Build history of the part. All positions in model axes, mm. Face numbers are marked on the shaded views. A direction names the side the tool comes from. Round coordinates to 2 decimals unless told otherwise and drop trailing zeros. Order: outer loops, then holes, each group sorted by start corner. A loop starts at its lowest first (then second) coordinate and runs counter-clockwise, first axis right, second up. Notation, with made-up numbers: M 88,54 L 94,54 A14 cw 94,71 Z; hole C 35.25,4.25 d2. An arc over 180 degrees is marked long. One line per item, written item: value. Start each with the question number.
Item 1: Pin check, flat tips, straight feed: pin 1 (1.5 mm diameter, centred on x = 0, y = -19, fed in from +Z) (3 decimals); pin 2 (1.3 mm diameter, centred on y = -19, z = 10.5, fed in from -X); pin 3 (3 mm diameter, centred on x = 4.5, y = 1.25, fed in from -Z); pin 4 (3.5 mm diameter, centred on y = -18.5, z = 7.5, fed in from +X). Stop position of each tip, or through.
Item 2: Band-saw the part on B-B, the plane x = 0. Write the cut outline in (y, z).
Item 3: Probe L1, parallel to Y at x = 0, z = 20; L2, parallel to X at y = 1.25, z = 12.25; L3, parallel to Y at x = -1, z = 7.25. List the from-to ranges inside material, lowest first.
Item 4: Band-saw the part on D-D, the plane z = 19. Write the cut outline in (x, y), then the cut area to 3 significant figures.
Item 5: Two-plate mould, pull along X, no slides. Class the marked faces 5, 6, 7 and 8: +X half, -X half, draft (parallel to the pull), parting line (faces both ways), or undercut.
Item 6: Band-saw the part on C-C, the plane y = 1.25. Write the cut outline in (x, z), then the cut area to 3 significant figures.
Item 7: Tool access for the marked faces 1, 2, 3 and 4: list every direction of +Z, -Z, +X, -X, +Y, -Y with a clear straight run to the whole face (end or side of a thin tool).
Item 8: Band-saw the part on A-A, the plane z = 16. Write the cut outline in (x, y), then the cut area to 3 significant figures.
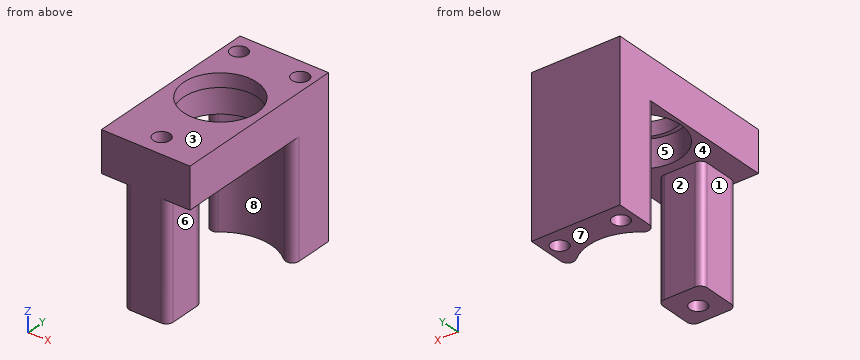
Autodesk Inventor part; units mm, degrees
ref_plane "YZ Plane" through (0, 0, 0) normal (1, 0, 0) x (0, 1, 0)
ref_plane "XZ Plane" through (0, 0, 0) normal (0, 1, 0) x (-1, 0, 0)
ref_plane "XY Plane" through (0, 0, 0) normal (0, 0, 1) x (1, 0, 0)
sketch "Sketch1" plane through (0, 0, 0) normal (0, 0, 1) x (1, 0, 0)
  line L0 (-6.5, 4) -> (6.5, 4)
  line L1 (6.5, 4) -> (6.5, -4)
  line L2 (6.5, -4) -> (-6.5, -4)
  line L3 (-6.5, -4) -> (-6.5, 4)
  line L4 (-6.5, 4) -> (6.5, -4) construction
  line L5 (6.5, 4) -> (-6.5, -4) construction
  point P0 (0, 0)
  point P1 (4.5, 1.25)
  point P2 (-4.5, 1.25)
  dimension "d0" = 13
  dimension "d1" = 8
  dimension "d64" = 2.75
  dimension "d65" = 2
  dimension "d66" = 2.75
  dimension "d67" = 2
extrude "Extrusion1" add sketch "Sketch1" along normal blind 48
hole "Hole1" at (-4.5, 1.25, 0) at (4.5, 1.25, 0) direction (0, 0, 1) diameter 2.459 end through all
sketch "Sketch6" plane through (-6.5, -4, 0) normal (0, -1, 0) x (1, 0, 0)
  line L0 (0.2, 0) -> (0, 0)
  line L1 (12.8, 0) -> (12.8, 36.9748)
  line L2 (0, 0) -> (12.8, 0)
  line L3 (12.8, 0) -> (12.8, 17)
  line L4 (12.8, 17) -> (0, 17)
  line L5 (0, 17) -> (0, 0)
  line L6 (13, 0) -> (13, 48)
  line L7 (0, 17) -> (13, 17)
  line L8 (13, 17) -> (13, 23)
  line L9 (13, 23) -> (0, 23)
  line L10 (0, 23) -> (0, 17)
  point P0 (6.5, 0)
  point P1 (12.8, 36.8338)
  point P2 (13, 36.8338)
  point P3 (13, 37.0101)
  dimension "d60" = 17
  dimension "d61" = 6
extrude "Extrusion3" add sketch "Sketch6" along normal blind 18 contours L10 L9 L1 L4 | L1 L9 L6 L7
sketch "Sketch7" plane through (6.5, -4, 17) normal (0, 0, -1) x (-1, 0, 0)
  line L0 (13, 8) -> (0, 8)
  circle A0 centre (6.5, -4) radius 6
  point P0 (6.5, 4)
  dimension "d68" = 12
  dimension "d69" = 12
extrude "Extrusion4" cut sketch "Sketch7" against normal blind 4
sketch "Sketch8" plane through (6.5, -22, 17) normal (0, 0, -1) x (-1, 0, 0)
  circle A0 centre (6.5, 14) radius 6
  circle A1 centre (6.5, 14) radius 7.5
  point P0 (6.5, 22)
  dimension "d72" = 15
extrude "Extrusion5" cut sketch "Sketch8" along normal through all contours A0 | A1
sketch "Sketch9" plane through (0, -8, 21) normal (0, 0, -1) x (-1, 0, 0)
  circle A0 centre (0, 0) radius 5.4
  point P0 (0, 8)
  dimension "d75" = 10.8
extrude "Extrusion6" cut sketch "Sketch9" against normal up to surface (2 mm away)
sketch "Sketch10" plane through (6.5, -22, 17) normal (0, 0, -1) x (-1, 0, 0)
  line L0 (3.25, 6.5) -> (3.25, 0)
  line L1 (3.25, 0) -> (9.75, 0)
  line L2 (9.75, 0) -> (9.75, 6.5)
  line L3 (9.75, 6.5) -> (3.25, 6.5)
  line L4 (3.25, 6.5) -> (9.75, 0) construction
  line L5 (3.25, 0) -> (9.75, 6.5) construction
  circle A0 centre (6.5, 14) radius 6
  circle A1 centre (6.5, 14) radius 7.5
  point P0 (6.5, 22)
  point P1 (6.5, 3.25)
  dimension "d78" = 6.5
  dimension "d80" = 6.5
  dimension "d81" = 3.25
  dimension "d95" = 7.5
extrude "Extrusion7" add sketch "Sketch10" along normal up to surface (17 mm away) contours L3 L2 L1 L0
sketch "Sketch11" plane through (3.25, -15.5, 0) normal (0, 0, -1) x (-1, 0, 0)
  line L0 (9.75, 19.5) -> (-3.25, 19.5)
  line L1 (-3.25, 19.5) -> (-3.25, 11.5)
  line L2 (6.5, 0) -> (0, 0)
  point P0 (3.25, 15.5)
  point P1 (3.25, -3.5)
  point P2 (9.55, 19.5)
  point P3 (-3.05, 19.5)
  point P4 (-3.25, 19.3)
  dimension "d85" = 6.5
  dimension "d96" = 3.5
  dimension "d97" = 23
hole "Hole5" at (0, -19, 0) direction (0, 0, 1) diameter 2.459 end through all
fillet "Fillet2" radius 1 8 edges at (-6.3443, -4, 8.5) (6.3443, -4, 8.5) (-6.5, -4, 8.5) (6.5, -4, 8.5) (-3.25, -15.5, 8.5) (3.25, -15.5, 8.5) (3.25, -22, 8.5) (-3.25, -22, 8.5)
sketch "Sketch13" plane through (0, 0, 0) normal (0, 0, -1) x (-1, 0, 0)
  point P0 (-4.5, 1.25)
move faces "Move1" translate (0, 0, -25) faces at (-1.2282, -2.5568, 48)
sketch "Sketch15" plane through (-6.5, -22, 23) normal (0, 0, 1) x (1, 0, 0)
  point P0 (6.5, 22)
properties part number "cam-flying-mount-rev2" material "Aluminum 6061"
Output:
1. pin 1: passes through
1. pin 2: stops at x = -3.25
1. pin 3: stops at z = 0
1. pin 4: stops at x = 3.25
2. outline: M -22,0 L -20.23,0 L -20.23,23 L -22,23 Z; M -17.77,0 L -15.5,0 L -15.5,17 L -14,17 L -14,21 L -13.4,21 L -13.4,23 L -17.77,23 Z; M -2.6,21 L -2,21 L -2,17 L -0.5,17 L -0.5,0 L 4,0 L 4,23 L -2.6,23 Z
3. L1: y = -22 to -20.23, -17.77 to -14, -2 to 4
3. L2: x = -6.5 to -5.73, -3.27 to 3.27, 5.73 to 6.5
3. L3: y = -22 to -19.72, -18.28 to -15.5, -0.57 to 4
4. outline: M -6.5,-22 L 6.5,-22 L 6.5,4 L -6.5,4 Z; hole C 0,-8 d12; hole C -4.5,1.25 d2.46; hole C 0,-19 d2.46; hole C 4.5,1.25 d2.46
4. area: 211 mm²
5. face 5: undercut
5. face 6: +X half
5. face 7: draft
5. face 8: undercut
6. outline: M -6.5,0 L -5.73,0 L -5.73,23 L -6.5,23 Z; M -3.27,0 L 3.27,0 L 3.27,23 L -3.27,23 Z; M 5.73,0 L 6.5,0 L 6.5,23 L 5.73,23 Z
6. area: 186 mm²
7. face 1: -Z, -X, -Y
7. face 2: -Z, +X, -X
7. face 3: +Z, +X, -X, +Y, -Y
7. face 4: -Z
8. outline: M -6.5,-1.52 A1 ccw -4.85,-2.28 A7.5 cw 4.85,-2.28 A1 ccw 6.5,-1.52 L 6.5,4 L -6.5,4 Z; M -3.25,-21 A1 ccw -2.25,-22 L 2.25,-22 A1 ccw 3.25,-21 L 3.25,-16.5 A1 ccw 2.25,-15.5 L -2.25,-15.5 A1 ccw -3.25,-16.5 Z; hole C -4.5,1.25 d2.46; hole C 0,-19 d2.46; hole C 4.5,1.25 d2.46
8. area: 97.2 mm²
